```python
from build123d import *

# Parameters (mm, degrees)
F0_W     = 12.8
F0_H     = 29
F1_DEPTH = 9
F2_W     = 12.8
F2_H     = 38
F3_DEPTH = 2
F4_W     = 12.8
F4_H     = 29
F5_DEPTH = 19
F7_D     = 4


with BuildPart() as f1:
    # F0 (on Front) → F1 (new body)
    with BuildSketch(Plane.XZ):
        Rectangle(F0_W, F0_H)
    extrude(amount=F1_DEPTH)

    # F2 (on face) → F3 (join)
    with BuildSketch(Plane(origin=(0, 0, 0), x_dir=(-1, 0, 0), z_dir=(0, 1, 0))):
        Rectangle(F2_W, F2_H)
    extrude(amount=-F3_DEPTH)

    # F4 (on face) → F5 (join)
    with BuildSketch(Plane(origin=(0, 0, 0), x_dir=(-1, 0, 0), z_dir=(0, 1, 0))):
        Rectangle(F4_W, F4_H)
    extrude(amount=F5_DEPTH)

    # F7 (through all)
    with Locations(Plane.XZ.offset(2)):
        with Locations((0, -17.5), (0, 17.5)):
            Hole(F7_D / 2)


solid = f1.part
```
Verification items for the finished model (mm, model axes). A direction names the side the tool comes from. Round coordinates to 2 decimals unless told otherwise and drop trailing zeros. Order: outer loops, then holes, each group sorted by start corner. A loop starts at its lowest first (then second) coordinate and runs counter-clockwise, first axis right, second up. Notation, with made-up numbers: (51, -8) - (80, -8) arc R29 ccw to (80, 17) - close; hole circle Ø6 at (-0.75, 59.5). An arc over 180 degrees is marked (long way). Use CSV: the item, a comma, the result in double quotes.
(1) Section check D-D on x = 0. Record the boundary of the cut face in (y, z), and give its area (3 significant figures).
Entries:
outline,"(-9, -14.5) - (-2, -14.5) - (-2, -15.5) - (0, -15.5) - (0, -14.5) - (19, -14.5) - (19, 14.5) - (0, 14.5) - (0, 15.5) - (-2, 15.5) - (-2, 14.5) - (-9, 14.5) - close"
area,"816 mm^2"
(2) Section check B-B on x = -4.5. Record the boundary of the cut face in (y, z), and give its area (3 significant figures).
Entries:
outline,"(-9, -14.5) - (-2, -14.5) - (-2, -19) - (0, -19) - (0, -14.5) - (19, -14.5) - (19, 14.5) - (0, 14.5) - (0, 19) - (-2, 19) - (-2, 14.5) - (-9, 14.5) - close"
area,"830 mm^2"
(3) Access from +Z, -Z, +X, -X, +Y, -Y to the whole of each face (thin tool, end or side, straight path). Record for faces 4 (the face through (0, 9, -14.5)), 5 (the face through (0, 0, 15)), 6 (the face through (0, -5, -14.5)).
Entries:
face 4,"-Z, +X, -X, +Y"
face 5,"+Z, +X, -X, +Y"
face 6,"-Z, +X, -X, -Y"
(4) Mould release check, pull along Z, two halves, no side actions. Record for faces 1 (the face through (0.07, -0.99, 15.5)), 2 (the face through (4, -1, -19)), 3 (the face through (0, 19, 0)): released by +Z, released by -Z, zero draft, split by the parting line, or undercut.
Entries:
face 1,"undercut"
face 2,"released by -Z"
face 3,"zero draft"
(5) Gauge pin test, flat ends, axial feed: pin 1 Ø1.3 at (x, z) = (1, 18) entering from -Y (1 decimal); pin 2 Ø1.3 at (x, z) = (3, 17) entering from +Y; pin 3 Ø5.5 at (x, y) = (1, -7) entering from -Z; pin 4 Ø4 at (x, y) = (3, 9.5) entering from +Z. Record the tip position at first contact, or that the pin passes through.
Entries:
pin 1,"through"
pin 2,"y = 0"
pin 3,"z = -14.5"
pin 4,"z = 14.5"
(6) Section check C-C on y = 15.25. Record the boundary of the cut face in (x, z), and give its area (3 significant figures).
Entries:
outline,"(-6.4, -14.5) - (6.4, -14.5) - (6.4, 14.5) - (-6.4, 14.5) - close"
area,"371 mm^2"
(7) Thickness scan on probe 1 along X at (y, z) = (-0.85, 17.5); probe 2 along Z at (x, y) = (0, -0.45); probe 3 along Y at (x, z) = (2, -15.5). Record the ranges inside material, lowest first. Write a range as from..to.
Entries:
probe 1,"-6.4..-2, 2..6.4"
probe 2,"-15.5..15.5"
probe 3,"-2..0"
(8) Section check A-A on z = -17.5. Record the boundary of the cut face in (x, y).
Entries:
outline,"(-6.4, -2) - (-2, -2) - (-2, 0) - (-6.4, 0) - close; (2, -2) - (6.4, -2) - (6.4, 0) - (2, 0) - close"
